```python
from build123d import *

# Parameters (mm, degrees)
F1_DEPTH = 5
F2_R     = 5
F3_DEPTH = 35
F4_R     = 5
F5_DEPTH = 6
F6_R     = 5
F7_DEPTH = 2


with BuildPart() as f1:
    # F0 (on Top) → F1 (new body)
    with BuildSketch(Plane.XY):
        Polygon((4.9074772881, 8.5), (-4.9074772881, 8.5), (-9.8149545762, 0), (-4.9074772881, -8.5), (4.9074772881, -8.5), (9.8149545762, 0), align=None)
    extrude(amount=F1_DEPTH)

    # F2 (on face) → F3 (join)
    with BuildSketch(Plane.XY.offset(5)):
        Circle(F2_R)
    extrude(amount=F3_DEPTH)

    # F4 (on face) → F5 (join)
    with BuildSketch(Plane.XY.offset(40)):
        Polygon((-8.5, 4.9074772881), (-8.5, -4.9074772881), (0, -9.8149545762), (8.5, -4.9074772881), (8.5, 4.9074772881), (0, 9.8149545762), align=None)
        Circle(F4_R, mode=Mode.SUBTRACT)
    extrude(amount=-F5_DEPTH)

    # F6 (on face) → F7 (cut)
    with BuildSketch(Plane.XY.offset(40)):
        Circle(F6_R)
    extrude(amount=-F7_DEPTH, mode=Mode.SUBTRACT)


solid = f1.part
```
The model under review builds one solid part; all positions refer to its coordinate system, in mm. A direction names the side the tool comes from. Coordinates: 2 decimals unless noted, no trailing zeros. Order: outer loops, then holes, each group sorted by start corner. A loop starts at its lowest first (then second) coordinate and runs counter-clockwise, first axis right, second up. Notation, with made-up numbers: (-2, 40.5) -> (28, 40.5) arc R21 cw to (28, 57.5) -> close; hole circle Ø5 at (35, -23.75). An arc over 180 degrees is marked (long way). Answer in a Markdown table with one row per item. Add a question column.
Item 1: To check wall thickness, follow probe 1 along Z at (x, y) = (-6.5, 1.5); probe 2 along Y at (x, z) = (0, 38.9); probe 3 along Z at (x, y) = (2.25, 1.5). State the ranges of each line that lie inside material, in increasing order.
Item 2: We need section A-A on y = 5.5. Write out the cut boundary in (x, z).
Item 3: We need section D-D on y = 2.75. Write out the cut boundary in (x, z).
Item 4: Mouldability with a two-part tool opening along Y and no side actions: class faces 1 (the cylindrical face through (-1.08, -4.88, 39.01)), 2 (the flat face through (4, -4, 34)), 3 (the flat face through (7.396, 4.19, 2.465)), 4 (the flat face through (4.19, -7.396, 37.042)) as +Y half, -Y half, draft (parallel to the pull), parting line (faces both ways), or undercut.
Item 5: Machinability: for faces 5 (the flat face through (0, 0, 38)), 6 (the flat face through (0, -8.5, 2)), 7 (the flat face through (0, 8.5, 2)), which of the approach directions +Z, -Z, +X, -X, +Y, -Y give a long, thin tool a straight path to every point of the face, cutting with its end or side? Answer none if there is none.
Item 6: We need section B-B on z = 36.5. Write out the cut boundary in (x, y), plus the area to 3 significant figures.
Item 7: We need section C-C on x = 2.75. Write out the cut boundary in (y, z), plus the area to 3 significant figures.
Item 8: Clearance check with flat-ended pins moving along their axes: pin 1 (3 mm diameter, centred on y = 0.5, z = 36, fed in from -X); pin 2 (6 mm diameter, centred on y = -6.5, z = 9, fed in from -X); pin 3 (9 mm diameter, centred on x = 0, y = 0, fed in from +Z); pin 4 (5 mm diameter, centred on x = 1.5, y = 2.5, fed in from -Z). State where each tip first meets the part, or that it passes through.
Final values:
| question | item | result |
|---|---|---|
| 1 | probe 1 | z = 0 to 5, 34 to 40 |
| 1 | probe 2 | y = -9.81 to -5, 5 to 9.81 |
| 1 | probe 3 | z = 0 to 38 |
| 2 | outline | (-7.47, 34) -> (7.47, 34) -> (7.47, 40) -> (-7.47, 40) -> close; (-6.64, 0) -> (6.64, 0) -> (6.64, 5) -> (-6.64, 5) -> close |
| 3 | outline | (-8.5, 34) -> (-4.18, 34) -> (-4.18, 5) -> (-8.23, 5) -> (-8.23, 0) -> (8.23, 0) -> (8.23, 5) -> (4.18, 5) -> (4.18, 34) -> (8.5, 34) -> (8.5, 40) -> (4.18, 40) -> (4.18, 38) -> (-4.18, 38) -> (-4.18, 40) -> (-8.5, 40) -> close |
| 4 | face 1 | undercut |
| 4 | face 2 | draft |
| 4 | face 3 | +Y half |
| 4 | face 4 | -Y half |
| 5 | face 5 | +Z |
| 5 | face 6 | -Z, +X, -X, -Y |
| 5 | face 7 | -Z, +X, -X, +Y |
| 6 | outline | (-8.5, -4.91) -> (0, -9.81) -> (8.5, -4.91) -> (8.5, 4.91) -> (0, 9.81) -> (-8.5, 4.91) -> close |
| 6 | area | 250 mm2 |
| 7 | outline | (-8.5, 0) -> (8.5, 0) -> (8.5, 5) -> (4.18, 5) -> (4.18, 34) -> (8.23, 34) -> (8.23, 40) -> (4.18, 40) -> (4.18, 38) -> (-4.18, 38) -> (-4.18, 40) -> (-8.23, 40) -> (-8.23, 34) -> (-4.18, 34) -> (-4.18, 5) -> (-8.5, 5) -> close |
| 7 | area | 409 mm2 |
| 8 | pin 1 | stops at x = -8.5 |
| 8 | pin 2 | stops at x = -3.57 |
| 8 | pin 3 | stops at z = 38 |
| 8 | pin 4 | stops at z = 0 |
